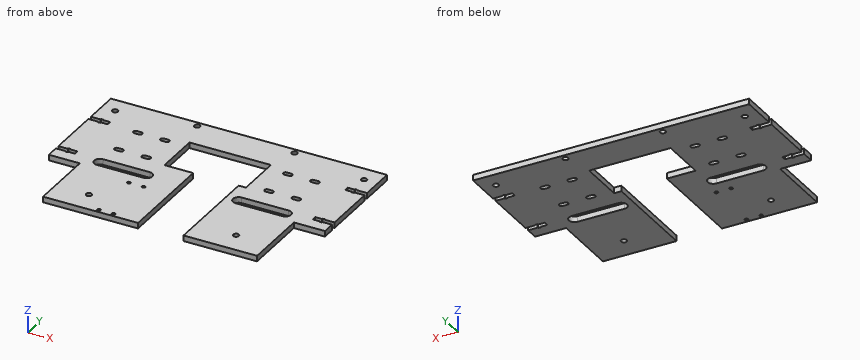
```python
from build123d import *

# Parameters (mm, degrees)
SKETCH1_W           = 244
SKETCH1_H           = 158.154567899
BOSS_EXTRUDE1_DEPTH = 5
SKETCH7_W           = 27.420299367
SKETCH7_H           = 58.920830548
SKETCH7_W_2         = 72
SKETCH7_H_2         = 40
CUT_EXTRUDE3_DEPTH  = 10
SKETCH8_W           = 40.15918936
SKETCH8_H           = 88.154567899
CUT_EXTRUDE4_DEPTH  = 10
SKETCH9_R           = 2.5
CUT_EXTRUDE5_DEPTH  = 10
CUT_EXTRUDE6_DEPTH  = 10
SKETCH13_R          = 1.5
CUT_EXTRUDE8_DEPTH  = 10
CUT_EXTRUDE10_DEPTH = 10
CUT_EXTRUDE11_DEPTH = 10


with BuildPart() as part:
    # Sketch1 → Boss-Extrude1 (new body)
    with BuildSketch(Plane.XY):
        with Locations((-158.307962763, -36.858709382)):
            Rectangle(SKETCH1_W, SKETCH1_H)
    extrude(amount=BOSS_EXTRUDE1_DEPTH)

    # Sketch7 → Cut-Extrude3 (cut)
    with BuildSketch(Plane(origin=(0, 0, 0), x_dir=(-1, 0, 0), z_dir=(0, 0, -1))):
        with Locations((266.59781308, -86.475578057)):
            Rectangle(SKETCH7_W, SKETCH7_H)
        with Locations((50.018112446, -86.475578057)):
            Rectangle(SKETCH7_W, SKETCH7_H)
        with Locations((158.307962763, -7.781425432)):
            Rectangle(SKETCH7_W_2, SKETCH7_H_2)
    extrude(amount=-CUT_EXTRUDE3_DEPTH, mode=Mode.SUBTRACT)

    # Sketch8 → Cut-Extrude4 (cut)
    with BuildSketch(Plane.XY.offset(5)):
        with Locations((-148.828368083, -71.858709382)):
            Rectangle(SKETCH8_W, SKETCH8_H)
    extrude(amount=-CUT_EXTRUDE4_DEPTH, mode=Mode.SUBTRACT)

    # Sketch9 → Cut-Extrude5 (cut)
    with BuildSketch(Plane.XY.offset(5)):
        with Locations((-93.307962763, -95.935993331)):
            Circle(SKETCH9_R)
        with Locations((-223.307962763, -95.935993331)):
            Circle(SKETCH9_R)
        with Locations((-268.307962763, 27.218574568)):
            Circle(SKETCH9_R)
        with Locations((-48.307962763, 27.218574568)):
            Circle(SKETCH9_R)
        with Locations((-115.307962763, 37.218574568)):
            Circle(SKETCH9_R)
        with Locations((-201.307962763, 37.218574568)):
            Circle(SKETCH9_R)
    extrude(amount=-CUT_EXTRUDE5_DEPTH, mode=Mode.SUBTRACT)

    # Sketch10 → Cut-Extrude6 (cut)
    with BuildSketch(Plane.XY.offset(5)):
        Polygon((-271.807962763, 10.218574568), (-280.307962763, 10.218574568), (-280.307962763, 6.218574568), (-271.807962763, 6.218574568), (-271.807962763, 5.466366238), (-269.407962763, 5.466366238), (-269.407962763, 6.218574568), (-263.307962763, 6.218574568), (-263.307962763, 10.218574568), (-269.407962763, 10.218574568), (-269.407962763, 10.968574568), (-271.807962763, 10.968574568), align=None)
        Polygon((-271.807962763, -41.781425432), (-280.307962763, -41.781425432), (-280.307962763, -45.781425432), (-271.807962763, -45.781425432), (-271.807962763, -46.531425432), (-269.407962763, -46.531425432), (-269.407962763, -45.781425432), (-263.307962763, -45.781425432), (-263.307962763, -41.781425432), (-269.407962763, -41.781425432), (-269.407962763, -41.029217101), (-271.807962763, -41.029217101), align=None)
        Polygon((-53.307962763, -41.781425432), (-53.307962763, -45.781425432), (-47.207962763, -45.781425432), (-47.207962763, -46.531425432), (-44.807962763, -46.531425432), (-44.807962763, -45.781425432), (-36.307962763, -45.781425432), (-36.307962763, -41.781425432), (-44.807962763, -41.781425432), (-44.807962763, -41.029217101), (-47.207962763, -41.029217101), (-47.207962763, -41.781425432), align=None)
        Polygon((-44.807962763, 6.218574568), (-36.307962763, 6.218574568), (-36.307962763, 10.218574568), (-44.807962763, 10.218574568), (-44.807962763, 10.968574568), (-47.207962763, 10.968574568), (-47.207962763, 10.218574568), (-53.307962763, 10.218574568), (-53.307962763, 6.218574568), (-47.207962763, 6.218574568), (-47.207962763, 5.466366238), (-44.807962763, 5.466366238), align=None)
    extrude(amount=-CUT_EXTRUDE6_DEPTH, mode=Mode.SUBTRACT)

    # Sketch13 → Cut-Extrude8 (cut)
    with BuildSketch(Plane.XY.offset(5)):
        with Locations((-205.205391913, -112.935993331)):
            Circle(SKETCH13_R)
        with Locations((-205.205391913, -64.935993331)):
            Circle(SKETCH13_R)
        with Locations((-192.205391913, -112.935993331)):
            Circle(SKETCH13_R)
        with Locations((-192.205391913, -64.935993331)):
            Circle(SKETCH13_R)
    extrude(amount=-CUT_EXTRUDE8_DEPTH, mode=Mode.SUBTRACT)

    # Sketch15 → Cut-Extrude10 (cut)
    with BuildSketch(Plane.XY.offset(5)):
        with BuildLine():
            Line((-198.907962763, -42.781425432), (-240.307962763, -42.781425432))
            ThreePointArc((-240.307962763, -42.781425432), (-245.307962763, -47.781425432), (-240.307962763, -52.781425432))
            Line((-240.307962763, -52.781425432), (-198.907962763, -52.781425432))
            ThreePointArc((-198.907962763, -52.781425432), (-193.907962763, -47.781425432), (-198.907962763, -42.781425432))
        make_face()
        with BuildLine():
            Line((-117.707962763, -42.781425432), (-76.307962763, -42.781425432))
            ThreePointArc((-76.307962763, -42.781425432), (-71.307962763, -47.781425432), (-76.307962763, -52.781425432))
            Line((-76.307962763, -52.781425432), (-117.707962763, -52.781425432))
            ThreePointArc((-117.707962763, -52.781425432), (-122.707962763, -47.781425432), (-117.707962763, -42.781425432))
        make_face()
    extrude(amount=-CUT_EXTRUDE10_DEPTH, mode=Mode.SUBTRACT)

    # Sketch16 → Cut-Extrude11 (cut)
    with BuildSketch(Plane.XY.offset(5)):
        with BuildLine():
            Line((-212.607962763, -25.881425432), (-210.607962763, -25.881425432))
            ThreePointArc((-210.607962763, -25.881425432), (-208.607962763, -23.881425432), (-210.607962763, -21.881425432))
            Line((-210.607962763, -21.881425432), (-214.607962763, -21.881425432))
            ThreePointArc((-214.607962763, -21.881425432), (-216.607962763, -23.881425432), (-214.607962763, -25.881425432))
            Line((-214.607962763, -25.881425432), (-212.607962763, -25.881425432))
        make_face()
        with BuildLine():
            Line((-236.607962763, -25.881425432), (-234.607962763, -25.881425432))
            ThreePointArc((-234.607962763, -25.881425432), (-232.607962763, -23.881425432), (-234.607962763, -21.881425432))
            Line((-234.607962763, -21.881425432), (-238.607962763, -21.881425432))
            ThreePointArc((-238.607962763, -21.881425432), (-240.607962763, -23.881425432), (-238.607962763, -25.881425432))
            Line((-238.607962763, -25.881425432), (-236.607962763, -25.881425432))
        make_face()
        with BuildLine():
            Line((-212.607962763, 4.118574568), (-210.607962763, 4.118574568))
            ThreePointArc((-210.607962763, 4.118574568), (-208.607962763, 6.118574568), (-210.607962763, 8.118574568))
            Line((-210.607962763, 8.118574568), (-212.607962763, 8.118574568))
            Line((-212.607962763, 8.118574568), (-214.607962763, 8.118574568))
            ThreePointArc((-214.607962763, 8.118574568), (-216.607962763, 6.118574568), (-214.607962763, 4.118574568))
            Line((-214.607962763, 4.118574568), (-212.607962763, 4.118574568))
        make_face()
        with BuildLine():
            Line((-236.607962763, 4.118574568), (-234.607962763, 4.118574568))
            ThreePointArc((-234.607962763, 4.118574568), (-232.607962763, 6.118574568), (-234.607962763, 8.118574568))
            Line((-234.607962763, 8.118574568), (-238.607962763, 8.118574568))
            ThreePointArc((-238.607962763, 8.118574568), (-240.607962763, 6.118574568), (-238.607962763, 4.118574568))
            Line((-238.607962763, 4.118574568), (-236.607962763, 4.118574568))
        make_face()
        with BuildLine():
            Line((-78.007962763, 4.118574568), (-80.007962763, 4.118574568))
            Line((-80.007962763, 4.118574568), (-82.007962763, 4.118574568))
            ThreePointArc((-82.007962763, 4.118574568), (-84.007962763, 6.118574568), (-82.007962763, 8.118574568))
            Line((-82.007962763, 8.118574568), (-78.007962763, 8.118574568))
            ThreePointArc((-78.007962763, 8.118574568), (-76.007962763, 6.118574568), (-78.007962763, 4.118574568))
        make_face()
        with BuildLine():
            Line((-78.007962763, -25.881425432), (-80.007962763, -25.881425432))
            Line((-80.007962763, -25.881425432), (-82.007962763, -25.881425432))
            ThreePointArc((-82.007962763, -25.881425432), (-84.007962763, -23.881425432), (-82.007962763, -21.881425432))
            Line((-82.007962763, -21.881425432), (-78.007962763, -21.881425432))
            ThreePointArc((-78.007962763, -21.881425432), (-76.007962763, -23.881425432), (-78.007962763, -25.881425432))
        make_face()
        with BuildLine():
            Line((-102.007962763, 8.118574568), (-104.007962763, 8.118574568))
            Line((-104.007962763, 8.118574568), (-106.007962763, 8.118574568))
            ThreePointArc((-106.007962763, 8.118574568), (-108.007962763, 6.118574568), (-106.007962763, 4.118574568))
            Line((-106.007962763, 4.118574568), (-104.007962763, 4.118574568))
            Line((-104.007962763, 4.118574568), (-102.007962763, 4.118574568))
            ThreePointArc((-102.007962763, 4.118574568), (-100.007962763, 6.118574568), (-102.007962763, 8.118574568))
        make_face()
        with BuildLine():
            Line((-102.007962763, -25.881425432), (-104.007962763, -25.881425432))
            Line((-104.007962763, -25.881425432), (-106.007962763, -25.881425432))
            ThreePointArc((-106.007962763, -25.881425432), (-108.007962763, -23.881425432), (-106.007962763, -21.881425432))
            Line((-106.007962763, -21.881425432), (-102.007962763, -21.881425432))
            ThreePointArc((-102.007962763, -21.881425432), (-100.007962763, -23.881425432), (-102.007962763, -25.881425432))
        make_face()
    extrude(amount=-CUT_EXTRUDE11_DEPTH, mode=Mode.SUBTRACT)


solid = part.part
```
Build history of the part. All positions in model axes, mm. Coordinates: 2 decimals unless noted, no trailing zeros. Write each loop counter-clockwise with the first axis right and the second up, starting at its lowest first coordinate (ties: lowest second). Pieces come first, ordered by that corner, then holes.
1. Band-saw the part on B-B, the plane x = -175. Give the cut face in (y, z).
Answer block:
outline: (-115.94, 0) - (-27.78, 0) - (-27.78, 5) - (-115.94, 5) - close; (12.22, 0) - (42.22, 0) - (42.22, 5) - (12.22, 5) - close
2. Band-saw the part on A-A, the plane y = -35. Give the cut face in (x, z).
Answer block:
outline: (-280.31, 0) - (-168.91, 0) - (-168.91, 5) - (-280.31, 5) - close; (-128.75, 0) - (-36.31, 0) - (-36.31, 5) - (-128.75, 5) - close
3. Band-saw the part on D-D, the plane z = 4.15. Give the number of separate pieces and of enclosed holes in the cut face, and give its area (3 significant figures).
Answer block:
separate pieces: 1
enclosed holes: 20
area: 27,300 mm2
4. Drill centre lines: probe 1 along Y at (x, z) = (-45.5, 2.7); probe 2 along Y at (x, z) = (-52, 0.6); probe 3 along Y at (x, z) = (-213.5, 1.9). Where is each one in solid material? Low to high.
Answer block:
probe 1: y = -57.02 to -46.53, -41.03 to 5.47, 10.97 to 42.22
probe 2: y = -57.02 to -45.78, -41.78 to 6.22, 10.22 to 42.22
probe 3: y = -115.94 to -52.78, -42.78 to -25.88, -21.88 to 4.12, 8.12 to 42.22
5. Drop a flat-ended pin along its axis: pin 1 (2.5 mm diameter, centred on x = -160.5, z = 1.5, fed in from -Y). Give the stop position or say it passes through.
Answer block:
pin 1: stops at y = 12.22
6. Band-saw the part on C-C, the plane x = -255.5. Give the cut face in (y, z).
Answer block:
outline: (-57.02, 0) - (42.22, 0) - (42.22, 5) - (-57.02, 5) - close
